Could you check a few things on this drawing? It's one solid part, dimensions in mm from its lowest x, y, z. A direction names the side the tool comes from. Give positions to 0.01 mm unless a question says otherwise; leave off trailing zeros. Loops run counter-clockwise (first coordinate to the right, second up) from the corner with the lowest first, then second, coordinate; pieces in that order, holes last. Notation, with made-up numbers: M 7.5,43 L 61.5,43 A18 cw 61.5,69 Z; hole C -9,68 d2. An arc over 180 degrees is marked long. Answer as a JSON object with one key per item and string values.
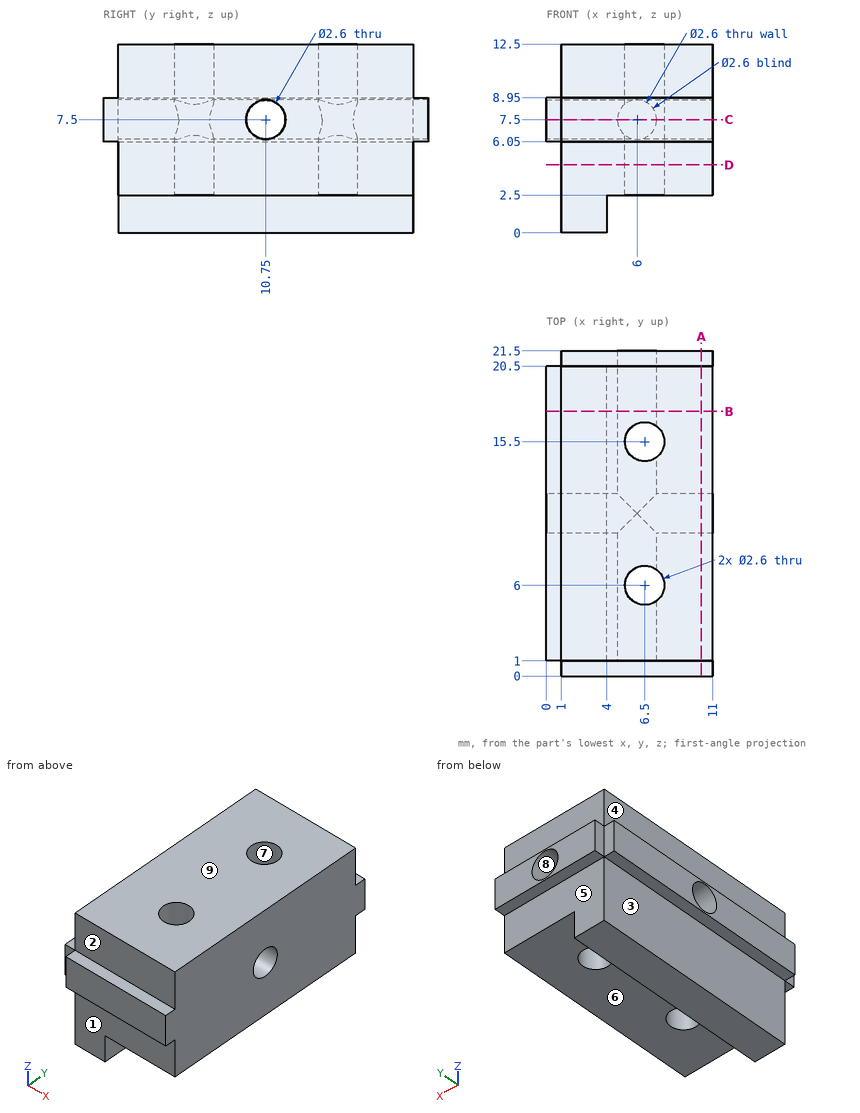
1) Suppose I cut it at D-D, the plane z = 4.5. Write out the boundary of the cut face in (x, y).
Answer list:
{"outline": "M 1,1 L 11,1 L 11,20.5 L 1,20.5 Z; hole C 6.5,6 d2.6; hole C 6.5,15.5 d2.6"}
2) For the marked faces 1, 2, 3, 4 and 5, which set-ups out of +Z, -Z, +X, -X, +Y, -Y let a thin tool reach every point of the face, with its end or its side?
Answer list:
{"face 1": "-Z, +X, -X, -Y", "face 2": "+Z, +X, -X, -Y", "face 3": "-Z, -X, +Y, -Y", "face 4": "+Z, -X, +Y, -Y", "face 5": "-Z, +X, -X, +Y"}
3) Suppose I cut it at C-C, the plane z = 7.5. Write out the boundary of the cut face in (x, y), and give its area (3 significant figures).
Answer list:
{"outline": "M 0,1 L 1,1 L 1,0 L 11,0 L 11,9.45 L 7.3,9.45 L 7.3,7.02 A1.3 cw 7.3,4.98 L 7.3,1 L 4.7,1 L 4.7,9.45 L 0,9.45 Z; M 0,12.05 L 4.7,12.05 L 4.7,21.5 L 1,21.5 L 1,20.5 L 0,20.5 Z; M 7.3,12.05 L 11,12.05 L 11,21.5 L 7.3,21.5 L 7.3,16.52 A1.3 cw 7.3,14.48 Z", "area": "158 mm^2"}
4) Please list where these lines run through material, in increasing order: line 1 along Y through (x, z) = (6.5, 5); line 2 along Y through (x, z) = (9.25, 7.5); line 3 along Y through (x, z) = (7.25, 6). Write a range as from..to.
Answer list:
{"line 1": "1..4.7, 7.3..14.2, 16.8..20.5", "line 2": "0..9.45, 12.05..21.5", "line 3": "1..4.94, 7.06..14.44, 16.56..20.5"}
5) Suppose I cut it at A-A, the plane x = 10.25. Write out the boundary of the cut face in (y, z).
Answer list:
{"outline": "M 0,6.05 L 1,6.05 L 1,2.5 L 20.5,2.5 L 20.5,6.05 L 21.5,6.05 L 21.5,8.95 L 20.5,8.95 L 20.5,12.5 L 1,12.5 L 1,8.95 L 0,8.95 Z; hole C 10.75,7.5 d2.6"}
6) Will these pins go through, and if not, where does the flat tip stop? pin 1 Ø1.8 at (y, z) = (14, 11) entering from -X; pin 2 Ø0.8 at (x, z) = (0.5, 7.5) entering from -Y; pin 3 Ø1.6 at (x, y) = (6.5, 15.5) entering from -Z; pin 4 Ø0.5 at (x, y) = (8, 21) entering from -Z.
Answer list:
{"pin 1": "x = 1", "pin 2": "y = 1", "pin 3": "through", "pin 4": "z = 6.05"}
7) If we mould it in two halves opening along Z, with no side actions, what happens to the marked faces 6, 7, 8 and 9? For each: +Z half, -Z half, draft (parallel to the pull), parting line (faces both ways), or undercut.
Answer list:
{"face 6": "-Z half", "face 7": "draft", "face 8": "undercut", "face 9": "+Z half"}
8) Suppose I cut it at B-B, the plane y = 17.5. Write out the boundary of the cut face in (x, z).
Answer list:
{"outline": "M 0,6.05 L 1,6.05 L 1,0 L 4,0 L 4,2.5 L 11,2.5 L 11,12.5 L 1,12.5 L 1,8.95 L 0,8.95 Z; hole C 6,7.5 d2.6"}
